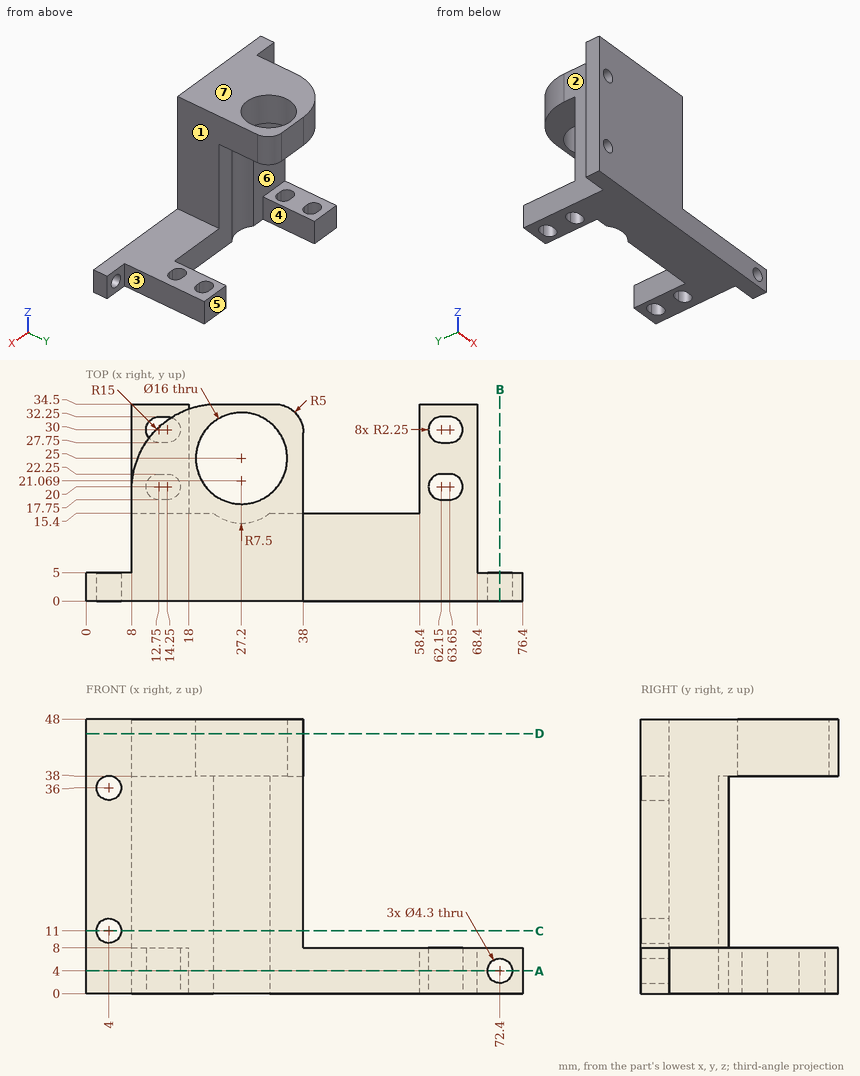
Part print with two shaded views. Sizes in mm from the minimum x, y, z corner. A direction names the side the tool comes from. Round coordinates to 2 decimals unless told otherwise and drop trailing zeros. Order: outer loops, then holes, each group sorted by start corner. A loop starts at its lowest first (then second) coordinate and runs counter-clockwise, first axis right, second up. Notation, with made-up numbers: M 63.25,73 L 104.25,73 A22 cw 104.25,112 Z; hole C 53.5,81 d7. An arc over 180 degrees is marked long. Put each result on its own line as item: value. Start each with the question number.
1. Slice it at C-C on z = 11. List the corners of the cut face in (x, y).
2. Slice it at B-B on x = 72.4. List the corners of the cut face in (y, z), then the cut area to 3 significant figures.
3. Slice it at A-A on z = 4. State how many separate pieces and enclosed holes the cut face has, then the cut area to 3 significant figures.
4. Two-plate mould, pull along Z, no slides. Class the marked faces 5, 6 and 7: +Z half, -Z half, draft (parallel to the pull), parting line (faces both ways), or undercut.
5. Drop flat-ended pins along their axis: pin 1 (1 mm diameter, centred on x = 21.5, z = 31, fed in from +Y); pin 2 (3 mm diameter, centred on y = 15.5, z = 29.5, fed in from +X); pin 3 (9 mm diameter, centred on y = 21.5, z = 5, fed in from +X); pin 4 (3.5 mm diameter, centred on x = 72.4, z = 4, fed in from +Y). Give the stop position or say it passes through.
6. Tool access for the marked faces 1, 2, 3 and 4: list every direction of +Z, -Z, +X, -X, +Y, -Y with a clear straight run to the whole face (end or side of a thin tool).
7. Drill centre lines: probe 1 along Z at (x, y) = (4, 2.4); probe 2 along X at (y, z) = (1, 11); probe 3 along X at (y, z) = (2, 4). Where is each one in solid material? Low to high. Write a range as [from, to].
8. Slice it at D-D on z = 45.5. List the corners of the cut face in (x, y), then the cut area to 3 significant figures.
Findings:
1. outline: M 0,0 L 1.85,0 L 1.85,5 L 0,5 Z; M 6.15,0 L 38,0 L 38,15.4 L 32.11,15.4 A7.5 cw 22.29,15.4 L 8,15.4 L 8,5 L 6.15,5 Z
2. outline: M 0,0 L 5,0 L 5,1.85 L 0,1.85 Z; M 0,6.15 L 5,6.15 L 5,8 L 0,8 Z
2. area: 18.5 mm2
3. separate pieces: 2
3. enclosed holes: 4
3. area: 1,270 mm2
4. face 5: draft
4. face 6: undercut
4. face 7: +Z half
5. pin 1: y = 15.4
5. pin 2: x = 38
5. pin 3: x = 68.4
5. pin 4: through
6. face 1: +Z, +X, +Y, -Y
6. face 2: +Z, -Z, -X, +Y
6. face 3: +Z, -Z, +X, +Y
6. face 4: -Z, +Y
7. probe 1: [0, 8.85], [13.15, 33.85], [38.15, 48]
7. probe 2: [0, 1.85], [6.15, 38]
7. probe 3: [0, 70.25], [74.55, 76.4]
8. outline: M 0,0 L 38,0 L 38,29.5 A5 ccw 33,34.5 L 23,34.5 A15 ccw 8,19.5 L 8,5 L 0,5 Z; hole C 27.2,25 d16
8. area: 820 mm2
